Source: CAD feature listing. Evaluate the final solid. Frame: model axes, mm. A direction names the side the tool comes from. Coordinates: 2 decimals unless noted, no trailing zeros. Order: outer loops, then holes, each group sorted by start corner. A loop starts at its lowest first (then second) coordinate and runs counter-clockwise, first axis right, second up. Notation, with made-up numbers: (-25.75, 81.5) -> (-2.75, 81.5) arc R8 cw to (-2.75, 90.5) -> close; hole circle Ø10 at (-33.75, 4). An arc over 180 degrees is marked (long way). Put each result on its own line as item: value.
from build123d import *

# Parameters (mm, degrees)
F0_R      = 15.875
F1_DEPTH  = 1016
F2_R      = 11.176
F3_DEPTH  = 1.8796
F4_R      = 10.3505
F5_DEPTH  = 76.2
F6_R      = 9.2583
F7_DEPTH  = 1016.001
F8_R      = 0.508
F9_R      = 15.875
F9_R_2    = 14.2875
F10_DEPTH = 30.48
F11_SIZE  = 1.016


with BuildPart() as f1:
    # F0 (on Front) → F1 (new body)
    with BuildSketch(Plane.XZ):
        Circle(F0_R)
    extrude(amount=F1_DEPTH)

    # F2 (on face) → F3 (cut)
    with BuildSketch(Plane.XZ.offset(1016)):
        Circle(F2_R)
    extrude(amount=-F3_DEPTH, mode=Mode.SUBTRACT)

    # F4 (on face) → F5 (cut)
    with BuildSketch(Plane.XZ.offset(1016)):
        Circle(F4_R)
    extrude(amount=-F5_DEPTH, mode=Mode.SUBTRACT)

    # F6 (on face) → F7 (cut, through all)
    with BuildSketch(Plane.XZ.offset(1016)):
        Circle(F6_R)
    extrude(amount=-F7_DEPTH, mode=Mode.SUBTRACT)

    # F8
    f8_edges = [f1.edges().sort_by_distance(p)[0] for p in [
        (-11.176, -1014.1204, 0),
    ]]
    fillet(f8_edges, radius=F8_R)

    # F9 (on face) → F10 (cut)
    with BuildSketch(Plane.XZ.offset(1016)):
        Circle(F9_R)
        Circle(F9_R_2, mode=Mode.SUBTRACT)
    extrude(amount=-F10_DEPTH, mode=Mode.SUBTRACT)

    # F11
    f11_edges = [f1.edges().sort_by_distance(p)[0] for p in [
        (-9.2583, -939.8, 0),
    ]]
    chamfer(f11_edges, length=F11_SIZE)


solid = f1.part
1. Set-up query: faces 1 (the cylindrical face through (-2.007, -475.963, -9.038)), 2 (the flat face through (-11.83, -985.52, 8.31)). Return all of +Z, -Z, +X, -X, +Y, -Y with unobstructed straight access to the full face (end or side cutting, diameter ignored); none if empty.
Numbers:
face 1: +Y, -Y
face 2: -Y
2. Pull-direction query (X, two-part tool) for faces 3 (the flat face through (-9, -1016, -7)), 4 (the cylindrical face through (-8.87, -1015.32, -6.8)), 5 (the cylindrical face through (-3.441, -485.861, -15.497)); classes: pulls with the +X half, pulls with the -X half, needs draft (parallel to the pull), parting line crosses it, or undercut.
Numbers:
face 3: needs draft
face 4: undercut
face 5: parting line crosses it
3. Ray query, line 1 along Z through (x, y) = (0, -997); line 2 along X through (y, z) = (-105.5, -1); line 3 along Z through (x, y) = (0, -731) (3 decimals). Return the intervals inside material, ascending.
Numbers:
line 1: z = -14.29 to -10.35, 10.35 to 14.29
line 2: x = -15.84 to -9.2, 9.2 to 15.84
line 3: z = -15.875 to -9.258, 9.258 to 15.875
4. Cut plane C-C on y = -166. Output: boundary loops of the cut face in (x, z) (3 decimals).
Numbers:
outline: circle Ø31.75 at (0, 0); hole circle Ø18.517 at (0, 0)
5. First-contact query: pin 1 (10.5 mm diameter, centred on x = -3.5, z = 3, fed in from -Y); pin 2 (12 mm diameter, centred on y = -667.5, z = 8.5, fed in from +X); pin 3 (1 mm diameter, centred on y = -522.5, z = 6.5, fed in from -X); pin 4 (6 mm diameter, centred on x = 1.5, z = 4, fed in from -Y). Flat tips, straight axial feed; report the tip coordinate or a pass-through.
Numbers:
pin 1: stops at y = -939.39
pin 2: stops at x = 15.68
pin 3: stops at x = -14.7
pin 4: passes through
